Verification items for the finished model (mm, model axes). A direction names the side the tool comes from. Give positions to 0.01 mm unless a question says otherwise; leave off trailing zeros. Write each loop counter-clockwise with the first axis right and the second up, starting at its lowest first coordinate (ties: lowest second). Pieces come first, ordered by that corner, then holes. Notation, with made-up numbers: (63.25, -17) -> (82.25, -17) arc R10 ccw to (82.25, 1) -> close; hole circle Ø9 at (6.25, -5). An arc over 180 degrees is marked (long way). Use CSV: the item, a comma, the result in double quotes. Start each with the question number.
```python
from build123d import *

# Parameters (mm, degrees)
F0_R     = 55
F0_R_2   = 51
F0_R_3   = 47
F1_DEPTH = 5
F2_DEPTH = 500
F3_DEPTH = 50
F4_R     = 7


with BuildPart() as f1:
    # F0 (on Top) → F1 (new body)
    with BuildSketch(Plane.XY):
        Circle(F0_R)
        Circle(F0_R_2, mode=Mode.SUBTRACT)
        Circle(F0_R_2)
        Circle(F0_R_3, mode=Mode.SUBTRACT)
        Circle(F0_R_3)
    extrude(amount=-F1_DEPTH)

    # F0 (on Top) → F2 (join)
    with BuildSketch(Plane.XY):
        Circle(F0_R_2)
        Circle(F0_R_3, mode=Mode.SUBTRACT)
    extrude(amount=F2_DEPTH)

    # F0 (on Top) → F3 (join)
    with BuildSketch(Plane.XY):
        Circle(F0_R)
        Circle(F0_R_2, mode=Mode.SUBTRACT)
    extrude(amount=F3_DEPTH)

    # F4
    f4_edges = [f1.edges().sort_by_distance(p)[0] for p in [
        (-55, 0, -5),
    ]]
    fillet(f4_edges, radius=F4_R)


solid = f1.part
```
(1) Section check A-A on z = 298. Record the cut outline in (x, y).
(2) Thickness scan on line 1 (Y direction, x = 0, z = 185); line 2 (Z direction, x = -8.5, y = 4.5); line 3 (Y direction, x = -6, z = 265.5). Record the ranges inside material, lowest first. Write a range as from..to.
(3) Draft check along Y on faces 1 (the face through (-11.056, -49.787, 271.85)), 2 (the face through (45, -15, 500)), 3 (the face through (-1, 1, 0)). Enter one of: released by +Y, released by -Y, zero draft, split by the parting line, or undercut.
(4) Set-up check for faces 4 (the face through (44.83, 14.12, 246.5)), 5 (the face through (-1, 1, -5)): record each of +Z, -Z, +X, -X, +Y, -Y from which the full face is reachable in a straight line by a thin tool's end or side.
(5) Go/stop test with flat-tipped pins: pin 1 (3 mm diameter, centred on y = -31, z = 358.5, fed in from -X); pin 2 (2 mm diameter, centred on x = -42, y = 0.5, fed in from +Z); pin 3 (6 mm diameter, centred on x = 22.5, z = 225, fed in from +Y). Record where each tip stops, or that it passes through.
Data:
1,outline,"circle Ø102 at (0, 0); hole circle Ø94 at (0, 0)"
2,line 1,"y = -51..-47, 47..51"
2,line 2,"z = -5..0"
2,line 3,"y = -50.65..-46.62, 46.62..50.65"
3,face 1,"split by the parting line"
3,face 2,"zero draft"
3,face 3,"undercut"
4,face 4,"+Z"
4,face 5,"-Z, +X, -X, +Y, -Y"
5,pin 1,"stops at x = -41.6"
5,pin 2,"stops at z = 0"
5,pin 3,"stops at y = 47.12"
